The listing builds one solid part. Answer for the finished solid, in the listing's coordinates (mm). A direction names the side the tool comes from. Give positions to 0.01 mm unless a question says otherwise; leave off trailing zeros. Loops run counter-clockwise (first coordinate to the right, second up) from the corner with the lowest first, then second, coordinate; pieces in that order, holes last. Notation, with made-up numbers: M -2.75,21 L 45.25,21 A21 ccw 45.25,32 Z; hole C 64.25,78.5 d8. An arc over 180 degrees is marked long. Return JSON: item names as keys, results as strings.
from build123d import *

# Parameters (mm, degrees)
SKETCH1_W               = 40
SKETCH1_H               = 60
BOSS_EXTRUDE1_DEPTH     = 100
CUT_EXTRUDE1_DEPTH      = 124.288280059
CUT_EXTRUDE1_DEPTH_BACK = 90
SKETCH2_W               = 34
SKETCH2_H               = 54
F_5_0_MM_DOWEL_HOLES1_D = 5


with BuildPart() as part:
    # Sketch1 → Boss-Extrude1 (new body)
    with BuildSketch(Plane(origin=(0, 0, 0), x_dir=(1, 0, 0), z_dir=(0, 1, 0))):
        with Locations((20, -30)):
            Rectangle(SKETCH1_W, SKETCH1_H)
    extrude(amount=BOSS_EXTRUDE1_DEPTH)

    # Sketch2 → Cut-Extrude1 (cut, two sides: drawn at the far end of the back side and taken through both)
    with BuildSketch(Plane(origin=(0, 100, 0), x_dir=(1, 0, 0), z_dir=(0, 1, 0)).offset(-CUT_EXTRUDE1_DEPTH_BACK)):
        with Locations((20, -30)):
            Rectangle(SKETCH2_W, SKETCH2_H)
    extrude(amount=CUT_EXTRUDE1_DEPTH + CUT_EXTRUDE1_DEPTH_BACK, mode=Mode.SUBTRACT)

    # Ø5.0 mm Dowel Holes1 (through all)
    with Locations(Plane(origin=(0, 10, 0), x_dir=(1, 0, 0), z_dir=(0, 1, 0))):
        with Locations((32.7, -12.22), (7.3, -12.22), (7.3, -47.78), (32.7, -47.78)):
            Hole(F_5_0_MM_DOWEL_HOLES1_D / 2)


solid = part.part
(1) Straight lines are drawn through the part: line 1 along X through (y, z) = (2, 12); line 2 along Z through (x, y) = (7.3, 7.75); line 3 along Z through (x, y) = (6, 67). For each, find the intervals that lie inside material, in ascending order.
Values follow:
{"line 1": "0 to 4.81, 9.79 to 30.21, 35.19 to 40", "line 2": "0 to 9.72, 14.72 to 45.28, 50.28 to 60", "line 3": "0 to 3, 57 to 60"}
(2) A tool of negligible diameter and unlimited length cuts with its end or side. For faces 1 (the flat face through (20, 10, 30)), 2 (the cylindrical face through (30.39, 4.93, 48.74)), from which of +Z, -Z, +X, -X, +Y, -Y can it reach the whole face along a straight path? Write none if from no direction.
Values follow:
{"face 1": "+Y", "face 2": "+Y, -Y"}
(3) The part is cut by section D-D (x = 24). Determine the outline of the cut face in (y, z), and give its area (3 significant figures).
Values follow:
{"outline": "M 0,0 L 100,0 L 100,3 L 10,3 L 10,57 L 100,57 L 100,60 L 0,60 Z", "area": "1,140 mm²"}
(4) The part is cut by section C-C (y = 33). Determine the outline of the cut face in (x, z), and give its area (3 significant figures).
Values follow:
{"outline": "M 0,0 L 40,0 L 40,60 L 0,60 Z; hole M 3,3 L 37,3 L 37,57 L 3,57 Z", "area": "564 mm²"}
(5) Determine the mould class of faces 3 (the flat face through (3, 54, 30)), 4 (the flat face through (20, 49, 0)), 5 (the cylindrical face through (30.315, 4.93, 11.469)), 6 (the flat face through (2, 100, 28)) for opening direction Z: released by +Z, released by -Z, zero draft, split by the parting line, or undercut.
Values follow:
{"face 3": "undercut", "face 4": "released by -Z", "face 5": "undercut", "face 6": "zero draft"}
(6) The part is cut by section B-B (x = 32.7). Determine the outline of the cut face in (y, z).
Values follow:
{"outline": "M 0,0 L 100,0 L 100,3 L 10,3 L 10,9.72 L 0,9.72 Z; M 0,14.72 L 10,14.72 L 10,45.28 L 0,45.28 Z; M 0,50.28 L 10,50.28 L 10,57 L 100,57 L 100,60 L 0,60 Z"}
(7) Given pin 1 (17 mm diameter, centred on x = 13, z = 32.5, fed in from +Y); pin 2 (3 mm diameter, centred on x = 32.7, z = 47.78, fed in from -Y), each flat-ended and moving along its own axis, determine where each tip first touches the part or whether it passes through.
Values follow:
{"pin 1": "y = 10", "pin 2": "through"}
(8) The part is cut by section A-A (z = 12.22). Determine the outline of the cut face in (x, y), and give its area (3 significant figures).
Values follow:
{"outline": "M 0,0 L 4.8,0 L 4.8,10 L 3,10 L 3,100 L 0,100 Z; M 9.8,0 L 30.2,0 L 30.2,10 L 9.8,10 Z; M 35.2,0 L 40,0 L 40,100 L 37,100 L 37,10 L 35.2,10 Z", "area": "840 mm²"}
